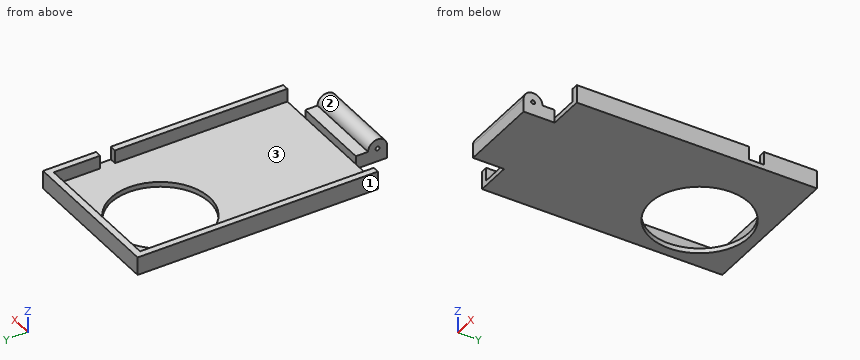
from build123d import *

# Parameters (mm, degrees)
F0_W      = 58.42
F0_H      = 92.71
F1_DEPTH  = 6.985
F2_W      = 53.34
F2_H      = 90.17
F3_DEPTH  = 5.08
F4_R      = 19.05
F5_DEPTH  = 25.4
F6_W      = 31.242
F6_H      = 12.0142
F7_DEPTH  = 5.08
F8_R      = 3.65125
F9_DEPTH  = 31.242
F10_R     = 0.762
F11_DEPTH = 38.1
F12_W     = 2.54
F12_H     = 5.715
F13_DEPTH = 5.08


with BuildPart() as f1:
    # F0 (on Top) → F1 (new body)
    with BuildSketch(Plane.XY):
        with Locations((5.7928592128, 9.0976799711)):
            Rectangle(F0_W, F0_H)
    extrude(amount=F1_DEPTH)

    # F2 (on face) → F3 (cut)
    with BuildSketch(Plane.XY.offset(6.985)):
        with Locations((5.7928592128, 7.8276799711)):
            Rectangle(F2_W, F2_H)
    extrude(amount=-F3_DEPTH, mode=Mode.SUBTRACT)

    # F4 (on face) → F5 (cut)
    with BuildSketch(Plane.XY.offset(1.905)):
        with Locations((-0.6841407872, 32.4656799711)):
            Circle(F4_R)
    extrude(amount=-F5_DEPTH, mode=Mode.SUBTRACT)

    # F6 (on face) → F7 (join)
    with BuildSketch(Plane(origin=(0, 0, 0), x_dir=(1, 0, 0), z_dir=(0, 0, -1))):
        with Locations((5.7928592128, 43.2644200289)):
            Rectangle(F6_W, F6_H)
    extrude(amount=-F7_DEPTH)

    # F8 (on face) → F9 (join)
    with BuildSketch(Plane(origin=(-9.8281407872, 0, 0), x_dir=(0, -1, 0), z_dir=(-1, 0, 0))):
        with Locations((45.6202700289, 5.08)):
            Circle(F8_R)
    extrude(amount=-F9_DEPTH)

    # F10 (on face) → F11 (cut)
    with BuildSketch(Plane(origin=(-9.8281407872, 0, 0), x_dir=(0, -1, 0), z_dir=(-1, 0, 0))):
        with Locations((45.6202700289, 5.08)):
            Circle(F10_R)
    extrude(amount=-F11_DEPTH, mode=Mode.SUBTRACT)

    # F12 (on face) → F13 (cut)
    with BuildSketch(Plane.XY.offset(6.985)):
        with Locations((33.7328592128, 32.1481799711)):
            Rectangle(F12_W, F12_H)
    extrude(amount=-F13_DEPTH, mode=Mode.SUBTRACT)


solid = f1.part
The model under review builds one solid part; all positions refer to its coordinate system, in mm. Face numbers are marked on the shaded views. Round coordinates to 2 decimals unless told otherwise and drop trailing zeros. Loops run counter-clockwise (first coordinate to the right, second up) from the corner with the lowest first, then second, coordinate; pieces in that order, holes last. Notation, with made-up numbers: (36, 57) -> (88, 57) arc R25 cw to (88, 82) -> close; hole circle Ø11 at (-2.5, 29.25). An arc over 180 degrees is marked (long way). Write item = value, one per line. Start each with the question number.
Item 1: To check wall thickness, follow L1, parallel to Y at x = 2.5, z = 2.5; L2, parallel to X at y = 38, z = 4.5; L3, parallel to Z at x = 22, y = -24 (3 decimals). State the ranges of each line that lie inside material, in increasing order.
Item 2: Take a section at A-A on x = 14.5. Give the boundary of the cut face in (y, z) (1 decimal).
Item 3: Take a section at C-C on x = -16.5. Give the boundary of the cut face in (y, z) (3 decimals).
Item 4: Take a section at D-D on x = 23. Give the boundary of the cut face in (y, z) (3 decimals).
Item 5: Take a section at B-B on y = 5. Give the boundary of the cut face in (x, z) (3 decimals).
Item 6: Insertion check: pin 1 (1.3 mm diameter, centred on x = 33.5, z = 5, fed in from -Y); pin 2 (3 mm diameter, centred on x = -9, y = -25, fed in from +Z) (3 decimals); pin 3 (2 mm diameter, centred on y = -45.62, z = 5.08, fed in from +X). Each pin has a flat end and moves straight along its axis. Give the tip position at first contact, or say it passes through.
Item 7: Mouldability with a two-part tool opening along Y and no side actions: class the marked faces 1, 2 and 3 as released by +Y, released by -Y, zero draft, split by the parting line, or undercut.
Result:
q1.L1 = -49.27 to -37.26, 52.91 to 55.45
q1.L2 = -23.42 to -20.88, 32.46 to 35
q1.L3 = 0 to 1.905
q2.outline = (-49.3, 0) -> (21, 0) -> (21, 1.9) -> (-37.3, 1.9) -> (-37.3, 5.1) -> (-42, 5.1) arc R3.7 ccw to (-49.3, 5.1) -> close; (44, 0) -> (55.5, 0) -> (55.5, 7) -> (52.9, 7) -> (52.9, 1.9) -> (44, 1.9) -> close; hole circle Ø1.5 at (-45.6, 5.1)
q3.outline = (-37.257, 0) -> (21.847, 0) -> (21.847, 1.905) -> (-37.257, 1.905) -> close; (43.085, 0) -> (55.453, 0) -> (55.453, 6.985) -> (52.913, 6.985) -> (52.913, 1.905) -> (43.085, 1.905) -> close
q4.outline = (-37.257, 0) -> (55.453, 0) -> (55.453, 6.985) -> (52.913, 6.985) -> (52.913, 1.905) -> (-37.257, 1.905) -> close
q5.outline = (-23.417, 0) -> (35.003, 0) -> (35.003, 6.985) -> (32.463, 6.985) -> (32.463, 1.905) -> (-20.877, 1.905) -> (-20.877, 6.985) -> (-23.417, 6.985) -> close
q6.pin_1 = -37.26
q6.pin_2 = 1.905
q6.pin_3 = 21.41
q7.face_1 = zero draft
q7.face_2 = undercut
q7.face_3 = undercut
